Autodesk Inventor part; units mm, degrees
ref_plane "YZ Plane" through (0, 0, 0) normal (1, 0, 0) x (0, 1, 0)
ref_plane "XZ Plane" through (0, 0, 0) normal (0, 1, 0) x (-1, 0, 0)
ref_plane "XY Plane" through (0, 0, 0) normal (0, 0, 1) x (1, 0, 0)
sketch "Sketch1" plane through (0, 0, 0) normal (0, 0, 1) x (1, 0, 0)
  line L0 (-12.1708, 16.0073) -> (13.2292, 16.0073)
  line L1 (13.2292, 16.0073) -> (13.2292, -34.7927)
  line L2 (13.2292, -34.7927) -> (-12.1708, -34.7927)
  line L3 (-12.1708, -34.7927) -> (-12.1708, 16.0073)
  line L4 (11.9592, 14.7373) -> (-10.9008, 14.7373)
  line L5 (-10.9008, 14.7373) -> (-10.9008, -33.5227)
  line L6 (-10.9008, -33.5227) -> (11.9592, -33.5227)
  line L7 (11.9592, -33.5227) -> (11.9592, 14.7373)
  point P0 (0, 0)
  dimension "d0" = 25.4
  dimension "d1" = 50.8
  dimension "d2" = 1.27
extrude "Extrusion1" add sketch "Sketch1" along normal blind 212.725
sketch "Sketch2" plane through (-12.1708, 16.0073, 0) normal (0, 1, 0) x (1, 0, 0)
  circle A0 centre (12.7, -12.7) radius 1.7272
  line L0 (25.4, 0) -> (0, 0)
  line L1 (0, 0) -> (0, -212.725)
  point P0 (12.1708, 0)
  dimension "d5" = 3.4544
  dimension "d6" = 12.7
  dimension "d7" = 12.7
extrude "Extrusion2" cut sketch "Sketch2" against normal through all
pattern_linear "Rectangular Pattern1" count 21 spacing 25.4 along (0, 0, 1) of "Extrusion2"
sketch "Sketch5" plane through (13.2292, -34.7927, 0) normal (1, 0, 0) x (0, 0, -1)
  line L0 (-212.725, 0) -> (-212.725, 50.8)
  line L1 (0, 50.8) -> (-212.725, 50.8)
  circle A0 centre (-28.575, 25.4) radius 14.2875
  line L2 (0, 0) -> (-212.725, 0)
  point P0 (0, 34.7927)
  dimension "d52" = 28.575
  dimension "d54" = 25.4
  dimension "d62" = 25.4
  dimension "d63" = 28.575
extrude "Extrusion5" cut sketch "Sketch5" against normal through all
equation "\"d3\" = d13"
equation "\"d10\" = d14"
equation "\"d13\" = 212.725"
equation "\"d14\" = d13"
equation "\"d32\" = 101.6"
properties part number "AIntakeSupport1"
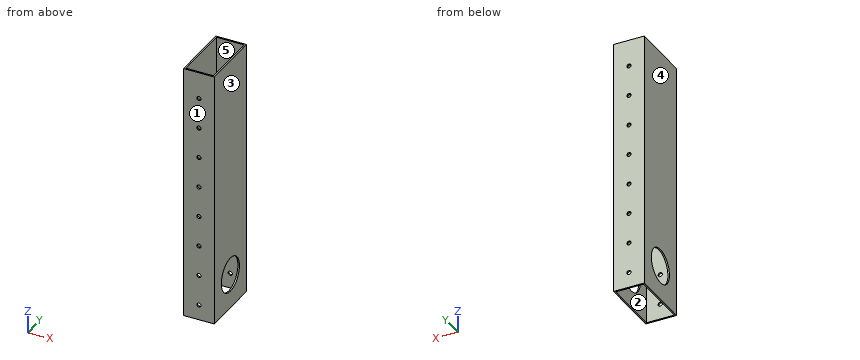
The model under review builds one solid part; all positions refer to its coordinate system, in mm. Face numbers are marked on the shaded views. A direction names the side the tool comes from. Coordinates: 2 decimals unless noted, no trailing zeros. Loops run counter-clockwise (first coordinate to the right, second up) from the corner with the lowest first, then second, coordinate; pieces in that order, holes last. Notation, with made-up numbers: (25.5, 38.25) -> (38.5, 38.25) arc R14 ccw to (38.5, 44.25) -> close; hole circle Ø1 at (46, 80.25). An arc over 180 degrees is marked (long way). Use a Markdown table: item, result. Add a question column.
1. Machinability: for the marked faces 4 and 5, which of the approach directions +Z, -Z, +X, -X, +Y, -Y give a long, thin tool a straight path to every point of the face, cutting with its end or side? Answer none if there is none.
2. Add section D-D on z = 19. Write out the cut boundary in (x, y), plus the area to 3 significant figures.
3. To check wall thickness, follow line 1 (X direction, y = -22, z = 73.5); line 2 (Y direction, x = -9.5, z = 61); line 3 (X direction, y = 15.55, z = 139.7). State the ranges of each line that lie inside material, in increasing order.
4. Clearance check with a flat-ended pin moving along its axis: pin 1 Ø4.5 at (x, z) = (0.53, 165.1) entering from +Y. State where the tip first meets the part, or that it passes through.
5. Add section C-C on y = -19. Write out the cut boundary in (x, z) (3 decimals), plus the area to 3 significant figures.
6. Add section A-A on x = -9. Write out the cut boundary in (y, z) (3 decimals), plus the area to 3 significant figures.
7. Draft analysis for pull direction Y (two halves, no side actions). For the marked faces 1, 2 and 3, state which applies: pulls with the +Y half, pulls with the -Y half, needs draft (parallel to the pull), parting line crosses it, or undercut.
8. Add section B-B on z = 105.5. Write out the cut boundary in (x, y).
Returned:
| question | item | result |
|---|---|---|
| 1 | face 4 | +Z, -Z, -X, +Y, -Y |
| 1 | face 5 | +Z, -Z |
| 2 | outline | (-12.17, -34.79) -> (13.23, -34.79) -> (13.23, -20) -> (11.96, -20) -> (11.96, -33.52) -> (-10.9, -33.52) -> (-10.9, -20) -> (-12.17, -20) -> close; (-12.17, 1.21) -> (-10.9, 1.21) -> (-10.9, 14.74) -> (11.96, 14.74) -> (11.96, 1.21) -> (13.23, 1.21) -> (13.23, 16.01) -> (-12.17, 16.01) -> close |
| 2 | area | 133 mm² |
| 3 | line 1 | x = -12.17 to -10.9, 11.96 to 13.23 |
| 3 | line 2 | y = -34.79 to -33.52, 14.74 to 16.01 |
| 3 | line 3 | x = -12.17 to -1.2, 2.26 to 13.23 |
| 4 | pin 1 | stops at y = 16.01 |
| 5 | outline | (-12.171, 0) -> (-10.901, 0) -> (-10.901, 18) -> (-12.171, 18) -> close; (-12.171, 39.15) -> (-10.901, 39.15) -> (-10.901, 212.725) -> (-12.171, 212.725) -> close; (11.959, 0) -> (13.229, 0) -> (13.229, 18) -> (11.959, 18) -> close; (11.959, 39.15) -> (13.229, 39.15) -> (13.229, 212.725) -> (11.959, 212.725) -> close |
| 5 | area | 487 mm² |
| 6 | outline | (-34.793, 0) -> (-33.523, 0) -> (-33.523, 212.725) -> (-34.793, 212.725) -> close; (14.737, 0) -> (16.007, 0) -> (16.007, 212.725) -> (14.737, 212.725) -> close |
| 6 | area | 540 mm² |
| 7 | face 1 | pulls with the -Y half |
| 7 | face 2 | undercut |
| 7 | face 3 | needs draft |
| 8 | outline | (-12.17, -34.79) -> (13.23, -34.79) -> (13.23, 16.01) -> (-12.17, 16.01) -> close; hole (-10.9, -33.52) -> (11.96, -33.52) -> (11.96, 14.74) -> (-10.9, 14.74) -> close |
